CAD build for the part. Positions are in the model's coordinates, mm. A direction names the side the tool comes from. Give positions to 0.01 mm unless a question says otherwise; leave off trailing zeros. Order: outer loops, then holes, each group sorted by start corner. A loop starts at its lowest first (then second) coordinate and runs counter-clockwise, first axis right, second up. Notation, with made-up numbers: M 61.25,15 L 67.25,15 A20 ccw 67.25,35 Z; hole C 2.25,-9 d3. An arc over 180 degrees is marked long. Put each result on its own line as item: value. Start each with the question number.
1) Two-plate mould, pull along Z, no slides. Class faces 1 (the face through (-0.33, -30.93, 2.52)), 2 (the face through (-41.275, 0, 0)), 3 (the face through (-38.02, -0.5, -2.23)), 4 (the face through (-29, 0, -3.175)): released by +Z, released by -Z, zero draft, split by the parting line, or undercut.
2) Pin check, flat tips, straight feed: pin 1 (1.5 mm diameter, centred on y = -1, z = 2.5, fed in from +X) (3 decimals); pin 2 (3 mm diameter, centred on x = 17, z = 0, fed in from -Y); pin 3 (1.5 mm diameter, centred on x = 0.5, z = -1, fed in from +Y) (3 decimals); pin 4 (2 mm diameter, centred on y = 22.5, z = -1, fed in from -X). Stop position of each tip, or through.
3) Cut at B-B (y = 25.5). Write the cut outline in (x, z) (3 decimals), and give its area (3 significant figures).
4) Cut at A-A (x = 0). Write the cut outline in (y, z) (1 decimal), and give its area (3 significant figures).
5) Tool access for faces 5 (the face through (-29, 0, 3.175)), 6 (the face through (38.11, -0.5, -2.23)), 7 (the face through (0, -33.338, 0)): list every direction of +Z, -Z, +X, -X, +Y, -Y with a clear straight run to the whole face (end or side of a thin tool).
6) Drill centre lines: line 1 (Z direction, x = 0, y = -31.5) (3 decimals); line 2 (Y direction, x = -0.5, z = -0.5); line 3 (Y direction, x = 2.5, z = -2). Where is each one in solid material? Low to high. Write a range as [from, to].
7) Cut at D-D (x = -32.5). Write the cut outline in (y, z) (3 decimals).
8) Cut at C-C (x = -15.5). Write the cut outline in (y, z) (3 decimals), and give its area (3 significant figures).
```python
from build123d import *

# Parameters (mm, degrees)
F0_R     = 34.925
F0_R_2   = 28.575
F1_DEPTH = 3.175
F2_R     = 2.286
F3_DEPTH = 41.275
F4_R     = 2.54
F5_DEPTH = 33.3375
F6_DEPTH = 12.7


with BuildPart() as f1:
    # F0 (on Top) → F1 (new body, symmetric)
    with BuildSketch(Plane.XY):
        Circle(F0_R)
        Circle(F0_R_2, mode=Mode.SUBTRACT)
    extrude(amount=F1_DEPTH, both=True)

    # F2 (on Right) → F3 (join, symmetric)
    with BuildSketch(Plane.YZ):
        Circle(F2_R)
    extrude(amount=F3_DEPTH, both=True)

    # F4 (on Front) → F5 (cut, symmetric)
    with BuildSketch(Plane.XZ):
        Circle(F4_R)
    extrude(amount=F5_DEPTH, both=True, mode=Mode.SUBTRACT)

    # F0 (on Top) → F6 (cut, symmetric)
    with BuildSketch(Plane.XY):
        Circle(F0_R_2)
    extrude(amount=F6_DEPTH, both=True, mode=Mode.SUBTRACT)


solid = f1.part
```
Solution:
1. face 1: undercut
1. face 2: zero draft
1. face 3: split by the parting line
1. face 4: released by -Z
2. pin 1: x = 41.275
2. pin 2: y = -31.3
2. pin 3: y = 34.925
2. pin 4: x = -27.52
3. outline: M -23.864,-3.175 L -12.895,-3.175 L -12.895,3.175 L -23.864,3.175 Z; M 12.895,-3.175 L 23.864,-3.175 L 23.864,3.175 L 12.895,3.175 Z
3. area: 139 mm²
4. outline: M -34.9,-3.2 L -28.6,-3.2 L -28.6,-2.5 L -33.3,-2.5 L -33.3,2.5 L -28.6,2.5 L -28.6,3.2 L -34.9,3.2 Z; M 28.6,-3.2 L 34.9,-3.2 L 34.9,3.2 L 28.6,3.2 L 28.6,2.5 L 33.3,2.5 L 33.3,-2.5 L 28.6,-2.5 Z
4. area: 32.3 mm²
5. face 5: +Z, +X, -X, +Y, -Y
5. face 6: +X
5. face 7: none
6. line 1: [-3.175, -2.54], [2.54, 3.175]
6. line 2: [-34.92, -33.34], [33.34, 34.92]
6. line 3: [-34.84, -28.47], [28.47, 34.84]
7. outline: M -12.787,-3.175 L 12.787,-3.175 L 12.787,3.175 L -12.787,3.175 Z
8. outline: M -31.297,-3.175 L -24.006,-3.175 L -24.006,3.175 L -31.297,3.175 Z; M 24.006,-3.175 L 31.297,-3.175 L 31.297,3.175 L 24.006,3.175 Z
8. area: 92.6 mm²
